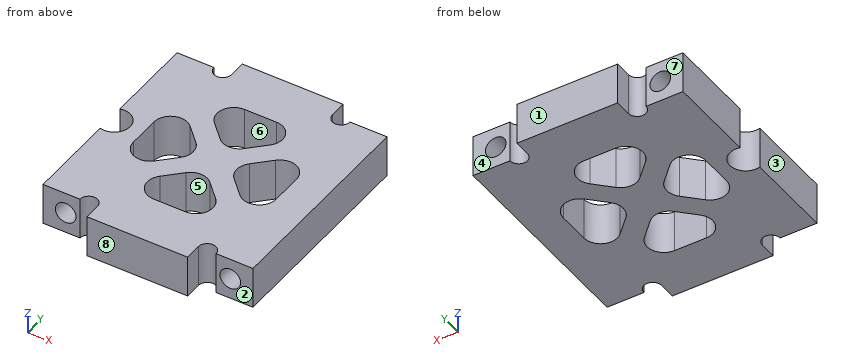
Autodesk Inventor part; units mm, degrees
ref_plane "YZ Plane" through (0, 0, 0) normal (1, 0, 0) x (0, 1, 0)
ref_plane "XZ Plane" through (0, 0, 0) normal (0, 1, 0) x (-1, 0, 0)
ref_plane "XY Plane" through (0, 0, 0) normal (0, 0, 1) x (1, 0, 0)
sketch "スケッチ1" plane through (0, 0, 0) normal (0, 0, 1) x (1, 0, 0)
  line L0 (-12.5, -12.5) -> (12.5, -12.5) construction
  line L1 (12.5, -12.5) -> (12.5, 12.5)
  line L2 (12.5, 12.5) -> (-12.5, 12.5) construction
  line L3 (-12.5, 12.5) -> (-12.5, -12.5)
  line L4 (-12.5, -12.5) -> (12.5, 12.5) construction
  line L5 (12.5, -12.5) -> (-12.5, 12.5) construction
  line L6 (-8.1, 12.5) -> (-12.5, 12.5)
  line L7 (8.1, 12.5) -> (12.5, 12.5)
  line L8 (-12.5, -12.5) -> (-8.1, -12.5)
  line L9 (8.1, -12.5) -> (12.5, -12.5)
  line L10 (-6, 12.5) -> (-6, 14.5)
  line L11 (-6, 14.5) -> (6, 14.5)
  line L12 (6, 14.5) -> (6, 12.5)
  arc A0 (-8.1, 12.5) -> (-6, 12.5) centre (-7.05, 12.5) ccw
  arc A1 (6, 12.5) -> (8.1, 12.5) centre (7.05, 12.5) ccw
  line L13 (0, 12.5) -> (0, 0) construction
  line L14 (0, 0) -> (12.5, 0) construction
  line L15 (-6, -12.5) -> (-6, -14.5)
  line L16 (-6, -14.5) -> (6, -14.5)
  line L17 (6, -14.5) -> (6, -12.5)
  arc A2 (-6, -12.5) -> (-8.1, -12.5) centre (-7.05, -12.5) ccw
  arc A3 (8.1, -12.5) -> (6, -12.5) centre (7.05, -12.5) ccw
  line L18 (-9.05, 12.5) -> (-5.95, 12.5) construction
  line L19 (-6.7322, 8.5) -> (6.7322, 8.5)
  line L20 (6.7322, 8.5) -> (0, 1.7678)
  line L21 (0, 1.7678) -> (-6.7322, 8.5)
  line L22 (-8.5, 6.7322) -> (-8.5, -6.7322)
  line L23 (-8.5, -6.7322) -> (-1.7678, 0)
  line L24 (-1.7678, 0) -> (-8.5, 6.7322)
  line L25 (-6.7322, -8.5) -> (6.7322, -8.5)
  line L26 (6.7322, -8.5) -> (0, -1.7678)
  line L27 (0, -1.7678) -> (-6.7322, -8.5)
  line L28 (8.5, 6.7322) -> (8.5, -6.7322)
  line L29 (8.5, -6.7322) -> (1.7678, 0)
  line L30 (1.7678, 0) -> (8.5, 6.7322)
  line L31 (12.5, 0) -> (12.3, 0)
  arc A4 (-12.5, -1.833) -> (-12.5, 1.833) centre (-12, 0) ccw
  point P0 (-12.5, 0)
  dimension "d0" = 25
  dimension "d1" = 1.05
  dimension "d2" = 2
  dimension "d3" = 6.5
  dimension "d9" = 2.5
  dimension "d10" = 2.5
  dimension "d11" = 2.5
  dimension "d12" = 2.5
  dimension "d13" = 4
  dimension "d31" = 25
  dimension "d44" = 1.9
  dimension "d46" = 0.5
extrude "押し出し1" add sketch "スケッチ1" along normal blind 2.5 contours L9 A3 L17 L16 L15 A2 L8 L3 A4 L6 A0 L10 L11 L12 A1 L7 L1
mirror "ミラー1" about plane through (0, 0, 0) normal (0, 0, -1) of "押し出し1"
sketch "スケッチ2" plane through (-12.5, -12.5, 2.5) normal (0, -1, 0) x (1, 0, 0)
  line L0 (6.5, 0) -> (18.5, 0) construction
  line L1 (12.5, 0) -> (12.5, -5) construction
  line L2 (0, -5) -> (4.4, -5)
  line L3 (20.6, -5) -> (25, -5)
  line L4 (0, -5) -> (0, 0)
  line L5 (25, -5) -> (25, 0)
  point P0 (12.5, -2.5)
  point P1 (2.7, -2.5)
  point P2 (22.3, -2.5)
  dimension "d35" = 2.5
  dimension "d37" = 2.5
  dimension "d47" = 2.7
  dimension "d48" = 2.7
hole "穴1" at (-9.8, -12.5, 0) at (9.8, -12.5, 0) direction (0, 1, 0) diameter 2.459 depth 8.8
pattern_circular "円形状パターン1" count 2 over 360 about axis through (0, 0, -10) along (0, 0, 1) of "穴1"
fillet "フィレット1" radius 2 12 edges at (8.5, 6.7322, 0) (8.5, -6.7322, 0) (6.7322, -8.5, 0) (0, 1.7678, 0) (-1.7678, 0, 0) (-6.7322, -8.5, 0) (-8.5, -6.7322, 0) (6.7322, 8.5, 0) (-8.5, 6.7322, 0) (-6.7322, 8.5, 0) (0, -1.7678, 0) (1.7678, 0, 0)
equation "\"d10\" = d9"
equation "\"d11\" = d10"
equation "\"d12\" = d11"
properties part number "Head_diagonal" material "アセタール樹脂、黒"
The listing builds one solid part. Answer for the finished solid, in the listing's coordinates (mm). Face numbers are marked on the shaded views. A direction names the side the tool comes from. Give positions to 0.01 mm unless a question says otherwise; leave off trailing zeros. Order: outer loops, then holes, each group sorted by start corner. A loop starts at its lowest first (then second) coordinate and runs counter-clockwise, first axis right, second up. Notation, with made-up numbers: (69.25, -24.5) -> (79.25, -24.5) arc R7 ccw to (79.25, -11.5) -> close; hole circle Ø4 at (-11.5, 6.25). An arc over 180 degrees is marked (long way). Put each result on its own line as item: value.
Item 1: A cutting plane is placed at A-A on y = 0. Give the vertices of the cut face in (x, z).
Established:
outline: (-10.1, -2.5) -> (-8.5, -2.5) -> (-8.5, 2.5) -> (-10.1, 2.5) -> close; (-2.6, -2.5) -> (2.6, -2.5) -> (2.6, 2.5) -> (-2.6, 2.5) -> close; (8.5, -2.5) -> (12.5, -2.5) -> (12.5, 2.5) -> (8.5, 2.5) -> close
Item 2: A cutting plane is placed at B-B on x = 0.75. Give the vertices of the cut face in (y, z), plus the area to 3 significant figures.
Established:
outline: (-14.5, -2.5) -> (-8.5, -2.5) -> (-8.5, 2.5) -> (-14.5, 2.5) -> close; (-2.74, -2.5) -> (2.74, -2.5) -> (2.74, 2.5) -> (-2.74, 2.5) -> close; (8.5, -2.5) -> (14.5, -2.5) -> (14.5, 2.5) -> (8.5, 2.5) -> close
area: 87.4 mm^2
Item 3: For the marked faces 1, 2, 3, 4 and 5, determine the directions among +Z, -Z, +X, -X, +Y, -Y from which every point of the face is accessible in a straight line to the end or side of a thin tool.
Established:
face 1: +Z, -Z, +X, -X, +Y
face 2: +Z, -Z, +X, -Y
face 3: +Z, -Z, -X, +Y, -Y
face 4: +Z, -Z, +X, +Y
face 5: +Z, -Z
Item 4: A cutting plane is placed at D-D on z = 0. Count the separate pieces of the cut face and the enclosed holes in it, plus the area to 3 significant figures.
Established:
separate pieces: 1
enclosed holes: 4
area: 434 mm^2
Item 5: Straight lines are drawn through the part: line 1 (X direction, y = 10.25, z = 0.05); line 2 (Y direction, x = -12, z = -0.45); line 3 (Z direction, x = 9.75, y = 9.75). For each, find the intervals that lie inside material, in ascending order.
Established:
line 1: x = -12.5 to -11.03, -8.57 to 8.57, 11.03 to 12.5
line 2: y = -12.5 to -1.9, 1.9 to 12.5
line 3: z = -2.5 to -1.23, 1.23 to 2.5
Item 6: For a pull along Y with two mould halves and no side action, classify the marked faces 6, 7 and 8 as released by +Y, released by -Y, zero draft, split by the parting line, or undercut.
Established:
face 6: undercut
face 7: released by +Y
face 8: released by -Y
Item 7: A cutting plane is placed at C-C on x = -5.5. Give the vertices of the cut face in (y, z), plus the area to 3 significant figures.
Established:
outline: (-14.5, -2.5) -> (-3.64, -2.5) -> (-3.64, 2.5) -> (-14.5, 2.5) -> close; (3.64, -2.5) -> (14.5, -2.5) -> (14.5, 2.5) -> (3.64, 2.5) -> close
area: 109 mm^2
Item 8: Given P1, Ø1.5, axis at y = -0.5, z = 0.5, coming from the -X side; P2, Ø1.5, axis at x = -9.8, z = 0, coming from the +Y side; P3, Ø1.6, axis at y = 14, z = -1, coming from the -X side; P4, Ø3, axis at x = 7, z = -2, coming from the -Y side, each flat-ended and moving along its own axis, determine where each tip first touches the part or whether it passes through.
Established:
P1: stops at x = -10.57
P2: stops at y = 3.7
P3: stops at x = -6
P4: stops at y = -14.5
